Source: CAD feature listing. Evaluate the final solid. Frame: model axes, mm. A direction names the side the tool comes from. Give positions to 0.01 mm unless a question says otherwise; leave off trailing zeros. Loops run counter-clockwise (first coordinate to the right, second up) from the corner with the lowest first, then second, coordinate; pieces in that order, holes last. Notation, with made-up numbers: (42.25, 4.25) -> (77.25, 4.25) arc R23 cw to (77.25, 39.25) -> close; hole circle Ø1 at (80.5, -30.5). An arc over 180 degrees is marked (long way). Return JSON: item names as keys, results as strings. Group by question number.
```python
from build123d import *

# Parameters (mm, degrees)
ESQUISSE1_W          = 14
ESQUISSE1_H          = 16.9
BASE_EXTRUSION_DEPTH = 9
EXTRUSION1_DEPTH     = 0.9
EXTRUSION2_DEPTH     = 0.9
ESQUISSE6_R          = 1.5
EXTRUSION3_DEPTH     = 7.7
EXTRUSION3_TAPER     = 3
CONG_1_R             = 1


with BuildPart() as part:
    # Esquisse1 → Base-Extrusion (new body)
    with BuildSketch(Plane.XY):
        with Locations((7, 8.45)):
            Rectangle(ESQUISSE1_W, ESQUISSE1_H)
    extrude(amount=BASE_EXTRUSION_DEPTH)

    # Esquisse4 → Extrusion1 (add)
    with BuildSketch(Plane.ZY):
        Polygon((3.607457233, 13.98057371), (-1.5, 13.98057371), (-1.5, 13.53057371), (-4, 13.53057371), (-4, 12.93057371), (-1.5, 12.93057371), (-1.5, 12.48057371), (3.607457233, 12.48057371), align=None)
        Polygon((3.607457233, 10.68057371), (-1.5, 10.68057371), (-1.5, 10.23057371), (-4, 10.23057371), (-4, 9.63057371), (-1.5, 9.63057371), (-1.5, 9.18057371), (3.607457233, 9.18057371), align=None)
        Polygon((3.607457233, 7.38057371), (-1.5, 7.38057371), (-1.5, 6.93057371), (-4, 6.93057371), (-4, 6.33057371), (-1.5, 6.33057371), (-1.5, 5.88057371), (3.607457233, 5.88057371), align=None)
        Polygon((3.607457233, 4.08057371), (-1.5, 4.08057371), (-1.5, 3.63057371), (-4, 3.63057371), (-4, 3.03057371), (-1.5, 3.03057371), (-1.5, 2.58057371), (3.607457233, 2.58057371), align=None)
    extrude(amount=EXTRUSION1_DEPTH)

    # Esquisse5 → Extrusion2 (add)
    with BuildSketch(Plane(origin=(14, 0, 0), x_dir=(0, 0, -1), z_dir=(1, 0, 0))):
        Polygon((1.5, 13.98057371), (-3.607457233, 13.98057371), (-3.607457233, 12.48057371), (1.5, 12.48057371), (1.5, 12.93057371), (4, 12.93057371), (4, 13.53057371), (1.5, 13.53057371), align=None)
        Polygon((1.5, 7.38057371), (-3.607457233, 7.38057371), (-3.607457233, 5.88057371), (1.5, 5.88057371), (1.5, 6.33057371), (4, 6.33057371), (4, 6.93057371), (1.5, 6.93057371), align=None)
        Polygon((-3.607457233, 10.68057371), (-3.607457233, 9.18057371), (1.5, 9.18057371), (1.5, 9.63057371), (4, 9.63057371), (4, 10.23057371), (1.5, 10.23057371), (1.5, 10.68057371), align=None)
        Polygon((-3.607457233, 4.08057371), (-3.607457233, 2.58057371), (1.5, 2.58057371), (1.5, 3.03057371), (4, 3.03057371), (4, 3.63057371), (1.5, 3.63057371), (1.5, 4.08057371), align=None)
    extrude(amount=EXTRUSION2_DEPTH)

    # Esquisse6 → Extrusion3 (add)
    with BuildSketch(Plane.XY.offset(9)):
        with Locations((7, 8.45)):
            Circle(ESQUISSE6_R)
    extrude(amount=EXTRUSION3_DEPTH, taper=EXTRUSION3_TAPER)

    # Congé1
    cong_1_edges = [part.edges().sort_by_distance(p)[0] for p in [
        (5.5, 8.45, 9),
    ]]
    fillet(cong_1_edges, radius=CONG_1_R)


solid = part.part
```
1) Contact query for flat-ended pins moving along their axis: P1, Ø0.7, axis at x = 14.5, z = -3, coming from the -Y side; P2, Ø4, axis at x = 13, y = 13.5, coming from the +Z side; P3, Ø0.7, axis at x = 14.5, z = -3, coming from the +Y side; P4, Ø4, axis at y = 4.5, z = 12.5, coming from the -X side. Output: stop coordinate, or through.
2) Cut plane D-D on z = 6.5. Return loops of the section in (x, y).
3) Mould query, pull axis Y, two halves, no side actions, for faces 6 (the face through (14.4, 12.931, -2.7)), 7 (the face through (14.4, 9.631, -2.7)), 8 (the face through (6.063, 9.309, 13.371)), 9 (the face through (7, 16.9, 4)). Classes: released by +Y, released by -Y, zero draft, split by the parting line, or undercut.
4) Cut plane A-A on z = -0.75. Count the separate pieces of the cut face and the enclosed holes in it, then the cut area to 3 significant figures.
5) Reachability of faces 1 (the face through (-0.4, 4.081, 1.1)), 2 (the face through (14.4, 7.381, 1)), 3 (the face through (14, 13.2, -1.5)), 4 (the face through (-0.4, 12.931, -2.8)), 5 (the face through (-0.4, 13.531, -2.7)) from +Z, -Z, +X, -X, +Y, -Y: full face, straight path, thin tool, end or side. Return the list, or none.
6) Cut plane C-C on x = 7. Return loops of the section in (y, z).
7) Cut plane B-B on y = 8.45. Return loops of the section in (x, z), then the cut area to 3 significant figures.
8) Material intervals for line 1 (X direction, y = 13, z = -1); line 2 (Z direction, x = 4.25, y = 7.25); line 3 (X direction, y = 5.75, z = 8), sorted ascending.
Calculated:
{
 "1": {"P1": "y = 3.03", "P2": "z = 9", "P3": "y = 13.53", "P4": "through"},
 "2": {"outline": "(0, 0) -> (14, 0) -> (14, 16.9) -> (0, 16.9) -> close"},
 "3": {"face 6": "undercut", "face 7": "undercut", "face 8": "split by the parting line", "face 9": "released by +Y"},
 "4": {"separate pieces": "8", "enclosed holes": "0", "area": "10.8 mm2"},
 "5": {"face 1": "+Z, -Z, -X", "face 2": "+Z, -Z, +X", "face 3": "-Z, +Y, -Y", "face 4": "-Z, +X, -X", "face 5": "-Z, +X, -X, +Y"},
 "6": {"outline": "(0, 0) -> (16.9, 0) -> (16.9, 9) -> (10.9, 9) arc R1 cw to (9.9, 9.95) -> (9.55, 16.7) -> (7.35, 16.7) -> (7, 9.95) arc R1 cw to (6, 9) -> (0, 9) -> close"},
 "7": {"outline": "(0, 0) -> (14, 0) -> (14, 9) -> (9.45, 9) arc R1 cw to (8.45, 9.95) -> (8.1, 16.7) -> (5.9, 16.7) -> (5.55, 9.95) arc R1 cw to (4.55, 9) -> (0, 9) -> close", "area": "146 mm2"},
 "8": {"line 1": "-0.9 to 0, 14 to 14.9", "line 2": "0 to 9", "line 3": "0 to 14"}
}
